Study the drawing (mm; zero at the part's minimum x, y, z) and answer. A direction names the side the tool comes from. Coordinates: 2 decimals unless noted, no trailing zeros. Write each loop counter-clockwise with the first axis right and the second up, starting at its lowest first coordinate (ties: lowest second). Pieces come first, ordered by that corner, then holes. Notation, with made-up numbers: M -27,-10.5 L 18,-10.5 A25 cw 18,22.5 Z; hole C -16,38.25 d10. An arc over 180 degrees is marked long. Answer as CSV lines item,"result". Start each with the question number.
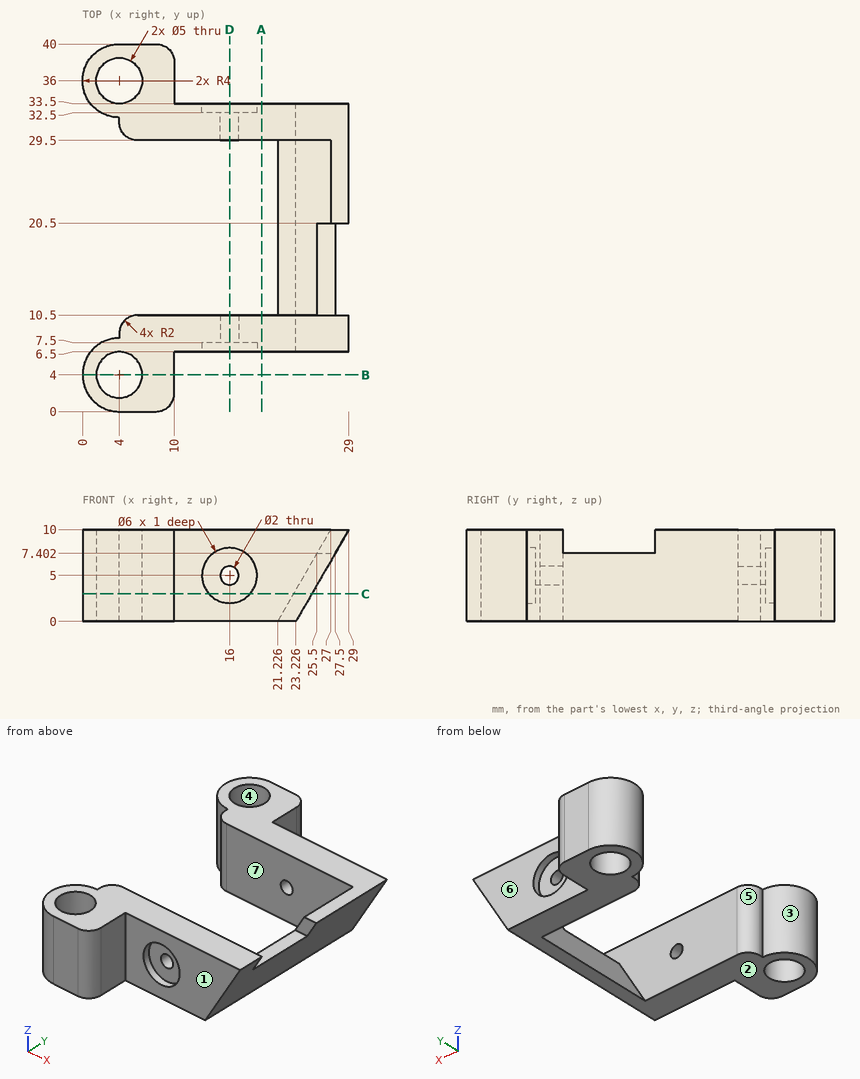
1) Which of the six approach directions +Z, -Z, +X, -X, +Y, -Y give full straight-line access (tool end or side, diameter ignored) to the marked faces 5, 6 and 7?
2) The part is cut by section D-D (x = 16). Determine the outline of the cut face in (y, z).
3) Each of these flat-tipped pins is pushed along its axis until it touches: P1, Ø4, axis at y = 22.5, z = 5.5, coming from the -X side; P2, Ø5, axis at x = 18.5, z = 7, coming from the +Y side; P3, Ø0.6, axis at x = 26.5, y = 14, coming from the +Z side. Where does it stop, or does it pass through?
4) For a pull along Y with two mould halves and no side action, classify the marked faces 1, 2, 3 and 4 as +Y half, -Y half, draft (parallel to the pull), parting line (faces both ways), or undercut.
5) The part is cut by section C-C (z = 3). Determine the outline of the cut face in (x, y), then the cut area to 3 significant figures.
6) The part is cut by section A-A (x = 19.5). Determine the outline of the cut face in (y, z).
7) Find the intervals of material crossed by line 1 (Y direction, x = 3.75, z = 4); line 2 (Y direction, x = 2.5, z = 6.5); line 3 (Y direction, x = 18.5, z = 4.75), in increasing order. Write a range as from..to.
8) The part is cut by section B-B (y = 4). Determine the outline of the cut face in (x, z), then the cut area to 3 significant figures.
Completed:
1,face 5,"+Z, -Z, -X"
1,face 6,"+Z, -Z, +X, +Y"
1,face 7,"+Z, -X"
2,outline,"M 6.5,0 L 10.5,0 L 10.5,4 L 7.5,4 L 7.5,2 L 6.5,2 Z; M 6.5,8 L 7.5,8 L 7.5,6 L 10.5,6 L 10.5,10 L 6.5,10 Z; M 29.5,0 L 33.5,0 L 33.5,2 L 32.5,2 L 32.5,4 L 29.5,4 Z; M 29.5,6 L 32.5,6 L 32.5,8 L 33.5,8 L 33.5,10 L 29.5,10 Z"
3,P1,"x = 23.25"
3,P2,"y = 33.5"
3,P3,"z = 7.4"
4,face 1,"-Y half"
4,face 2,"draft"
4,face 3,"undercut"
4,face 4,"undercut"
5,outline,"M 4,0 L 8,0 A2 ccw 10,2 L 10,6.5 L 13.76,6.5 L 13.76,7.5 L 18.24,7.5 L 18.24,6.5 L 24.96,6.5 L 24.96,33.5 L 18.24,33.5 L 18.24,32.5 L 13.76,32.5 L 13.76,33.5 L 10,33.5 L 10,38 A2 ccw 8,40 L 4,40 A4 ccw 4,32 L 4,31.5 A2 ccw 6,29.5 L 22.96,29.5 L 22.96,10.5 L 6,10.5 A2 ccw 4,8.5 L 4,8 A4 ccw Z; hole C 4,4 d5; hole C 4,36 d5"
5,area,"282 mm²"
6,outline,"M 6.5,0 L 10.5,0 L 10.5,10 L 6.5,10 Z; M 29.5,0 L 33.5,0 L 33.5,10 L 29.5,10 Z"
7,line 1,"0.01..1.51, 6.49..7.99, 32.01..33.51, 38.49..39.99"
7,line 2,"0.29..2, 6..7.71, 32.29..34, 38..39.71"
7,line 3,"7.5..10.5, 29.5..32.5"
8,outline,"M 0,0 L 1.5,0 L 1.5,10 L 0,10 Z; M 6.5,0 L 10,0 L 10,10 L 6.5,10 Z"
8,area,"50.0 mm²"
